The listing builds one solid part. Answer for the finished solid, in the listing's coordinates (mm). Face numbers are marked on the shaded views. A direction names the side the tool comes from. Give positions to 0.01 mm unless a question says otherwise; leave off trailing zeros. Order: outer loops, then holes, each group sorted by start corner. A loop starts at its lowest first (then second) coordinate and runs counter-clockwise, first axis right, second up. Notation, with made-up numbers: (19, -9.5) - (63, -9.5) arc R8 cw to (63, -1.5) - close; hole circle Ø1 at (56, -8). An arc over 180 degrees is marked (long way). Answer as a JSON object with one key per item and string values. Group by question number.
Q1. A cutting plane is placed at C-C, the plane x = 31.75. Give the vertices of the cut face in (y, z).
Q2. Given pin 1 (3 mm diameter, centred on y = 4.5, z = -9.5, fed in from -X); pin 2 (6.5 mm diameter, centred on x = 18.5, z = 2, fed in from +Y); pin 3 (5 mm diameter, centred on x = -24.5, z = -7, fed in from -Y); pin 4 (3.5 mm diameter, centred on x = -20.5, y = 0, fed in from -Z), each flat-ended and moving along its own axis, determine where each tip first touches the part or whether it passes through.
Q3. Consider line 1 (X direction, y = -0.65, z = 0) (1 decimal); line 2 (Y direction, x = 28, z = -2.5); line 3 (X direction, y = 9.5, z = -12.5). Determine where each line is inside the solid, lowest interval first.
Q4. For the marked faces 1, 2 and 3, determine the directions among +Z, -Z, +X, -X, +Y, -Y from which every point of the face is accessible in a straight line to the end or side of a thin tool.
Q5. A cutting plane is placed at A-A, the plane z = 0. Give the vertices of the cut face in (x, y) (1 decimal), and give its area (3 significant figures).
Q6. A cutting plane is placed at B-B, the plane y = 0.25. Count the separate pieces of the cut face and the enclosed holes in it, and give its area (3 significant figures).
Q7. The mould has two halves that part along Z. Classify the marked faces 4, 5 and 6: released by +Z, released by -Z, zero draft, split by the parting line, or undercut.
Q8. A cutting plane is placed at D-D, the plane x = -22.5. Give the vertices of the cut face in (y, z), and give its area (3 significant figures).
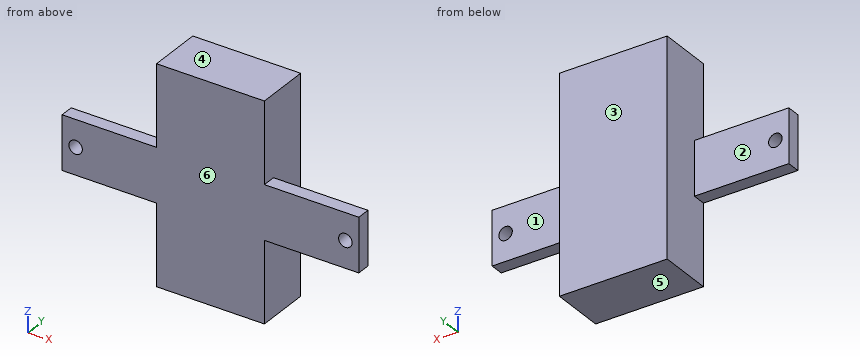
from build123d import *

# Parameters (mm, degrees)
SKETCH2_W           = 69.85
SKETCH2_H           = 3.175
BOSS_EXTRUDE1_DEPTH = 6.35
SKETCH5_W           = 25.4
SKETCH5_H           = 12.7
BOSS_EXTRUDE2_DEPTH = 25.4
SKETCH6_R           = 1.5875
CUT_EXTRUDE1_DEPTH  = 45.22263278


with BuildPart() as part:
    # Sketch2 → Boss-Extrude1 (new, symmetric)
    with BuildSketch(Plane.XY):
        Rectangle(SKETCH2_W, SKETCH2_H)
    extrude(amount=BOSS_EXTRUDE1_DEPTH, both=True)

    # Sketch5 → Boss-Extrude2 (add, symmetric)
    with BuildSketch(Plane.XY):
        with Locations((0, 4.7625)):
            Rectangle(SKETCH5_W, SKETCH5_H)
    extrude(amount=BOSS_EXTRUDE2_DEPTH, both=True)

    # Sketch6 → Cut-Extrude1 (cut, through all)
    with BuildSketch(Plane(origin=(0, 1.5875, 0), x_dir=(1, 0, 0), z_dir=(0, 1, 0))):
        with Locations(Location((-31.75, 0, 0), (0, 0, 270))):
            Circle(SKETCH6_R)
        with Locations(Location((31.75, 0, 0), (0, 0, 270))):
            Circle(SKETCH6_R)
    extrude(amount=-CUT_EXTRUDE1_DEPTH, mode=Mode.SUBTRACT)


solid = part.part
Reply:
{
 "1": {"outline": "(-1.59, -6.35) - (1.59, -6.35) - (1.59, -1.59) - (-1.59, -1.59) - close; (-1.59, 1.59) - (1.59, 1.59) - (1.59, 6.35) - (-1.59, 6.35) - close"},
 "2": {"pin 1": "stops at x = -12.7", "pin 2": "stops at y = 1.59", "pin 3": "stops at y = -1.59", "pin 4": "stops at z = -6.35"},
 "3": {"line 1": "x = -34.9 to -33.3, -30.2 to 30.2, 33.3 to 34.9", "line 2": "y = -1.59 to 1.59", "line 3": "x = -12.7 to 12.7"},
 "4": {"face 1": "+Z, -Z, +X, +Y", "face 2": "+Z, -Z, -X, +Y", "face 3": "+Z, -Z, +X, -X, +Y"},
 "5": {"outline": "(-34.9, -1.6) - (-33.3, -1.6) - (-33.3, 1.6) - (-34.9, 1.6) - close; (-30.2, -1.6) - (30.2, -1.6) - (30.2, 1.6) - (12.7, 1.6) - (12.7, 11.1) - (-12.7, 11.1) - (-12.7, 1.6) - (-30.2, 1.6) - close; (33.3, -1.6) - (34.9, -1.6) - (34.9, 1.6) - (33.3, 1.6) - close", "area": "444 mm^2"},
 "6": {"separate pieces": "1", "enclosed holes": "2", "area": "1,840 mm^2"},
 "7": {"face 4": "released by +Z", "face 5": "released by -Z", "face 6": "zero draft"},
 "8": {"outline": "(-1.59, -6.35) - (1.59, -6.35) - (1.59, 6.35) - (-1.59, 6.35) - close", "area": "40.3 mm^2"}
}
